from build123d import *

# Parameters (mm, degrees)
SKETCH_W        = 720
SKETCH_H        = 720
PAD_DEPTH       = 10
SKETCH001_W     = 700
SKETCH001_H     = 700
SKETCH001_W_2   = 680
SKETCH001_H_2   = 680
PAD001_DEPTH    = 50
SKETCH002_W     = 46
SKETCH002_H     = 40
SKETCH002_H_2   = 200
PAD002_DEPTH    = 10
SKETCH003_W     = 46
SKETCH003_H     = 61
PAD003_DEPTH    = 5
SKETCH004_W     = 132
SKETCH004_H     = 61
PAD004_DEPTH    = 46
POCKET_DEPTH    = 61
SKETCH006_R     = 2.5
PAD005_DEPTH    = 14
POCKET001_DEPTH = 10
SKETCH008_W     = 5
SKETCH008_H     = 83
SKETCH008_H_2   = 35
POCKET002_DEPTH = 10
FILLET_R        = 3
FILLET001_R     = 3
FILLET002_R     = 1
FILLET003_R     = 5
SKETCH009_W     = 80
SKETCH009_H     = 40
POCKET003_DEPTH = 10


with BuildPart() as part:
    # Sketch → Pad (new body)
    with BuildSketch(Plane.XY):
        Rectangle(SKETCH_W, SKETCH_H)
    extrude(amount=PAD_DEPTH)

    # Sketch001 (on Face5 of Pad) → Pad001 (join)
    with BuildSketch(Plane(origin=(0, 0, 0), x_dir=(1, 0, 0), z_dir=(0, 0, -1))):
        Rectangle(SKETCH001_W, SKETCH001_H)
        Rectangle(SKETCH001_W_2, SKETCH001_H_2, mode=Mode.SUBTRACT)
    extrude(amount=PAD001_DEPTH)

    # Sketch002 (on Face16 of Pad001) → Pad002 (join)
    with BuildSketch(Plane(origin=(0, 0, 0), x_dir=(1, 0, 0), z_dir=(0, 0, -1))):
        with Locations((282, -285)):
            Rectangle(SKETCH002_W, SKETCH002_H)
        with Locations((231, -285)):
            Rectangle(SKETCH002_W, SKETCH002_H)
        with Locations((282, -84)):
            Rectangle(SKETCH002_W, SKETCH002_H_2)
        with Locations((231, -84)):
            Rectangle(SKETCH002_W, SKETCH002_H_2)
    extrude(amount=PAD002_DEPTH)

    # Sketch003 (on Face16 of Pad002) → Pad003 (join)
    with BuildSketch(Plane(origin=(0, 0, 0), x_dir=(1, 0, 0), z_dir=(0, 0, -1))):
        with Locations((231, -224.5)):
            Rectangle(SKETCH003_W, SKETCH003_H)
        with Locations((282, -224.5)):
            Rectangle(SKETCH003_W, SKETCH003_H)
    extrude(amount=PAD003_DEPTH)

    # Sketch004 (on Face16 of Pad003) → Pad004 (join)
    with BuildSketch(Plane(origin=(0, 0, 0), x_dir=(1, 0, 0), z_dir=(0, 0, -1))):
        with Locations((-174, 209.5)):
            Rectangle(SKETCH004_W, SKETCH004_H)
    extrude(amount=PAD004_DEPTH)

    # Sketch005 (on Face42 of Pad004) → Pocket (cut)
    with BuildSketch(Plane(origin=(0, -179, 0), x_dir=(-1, 0, 0), z_dir=(0, 1, 0))):
        Polygon((108, -46), (240, -46), (179, 0), (169, 0), align=None)
    extrude(amount=-POCKET_DEPTH, mode=Mode.SUBTRACT)

    # Sketch006 (on Face16 of Pocket) → Pad005 (join)
    with BuildSketch(Plane(origin=(0, 0, 0), x_dir=(1, 0, 0), z_dir=(0, 0, -1))):
        with Locations((-241.5, -208.5)):
            Circle(SKETCH006_R)
    extrude(amount=PAD005_DEPTH)

    # Sketch007 (on Face13 of Pad005) → Pocket001 (cut)
    with BuildSketch(Plane.XZ.offset(-340)):
        with BuildLine():
            ThreePointArc((-292.75, -25), (-307.75, -10), (-322.75, -25))
            Line((-322.75, -50), (-322.75, -25))
            Line((-322.75, -50), (-292.75, -50))
            Line((-292.75, -50), (-292.75, -25))
        make_face()
    extrude(amount=-POCKET001_DEPTH, mode=Mode.SUBTRACT)

    # Sketch008 (on Face19 of Pocket001) → Pocket002 (cut)
    with BuildSketch(Plane(origin=(0, 0, 0), x_dir=(1, 0, 0), z_dir=(0, 0, -1))):
        with Locations((-286.5, -208.5)):
            Rectangle(SKETCH008_W, SKETCH008_H)
        with Locations((-279, -208.5)):
            Rectangle(SKETCH008_W, SKETCH008_H)
        with Locations((-271.5, -208.5)):
            Rectangle(SKETCH008_W, SKETCH008_H)
        with Locations((-264, -208.5)):
            Rectangle(SKETCH008_W, SKETCH008_H)
        with Locations((-256.5, -208.5)):
            Rectangle(SKETCH008_W, SKETCH008_H)
        with Locations((-249, -208.5)):
            Rectangle(SKETCH008_W, SKETCH008_H)
        with Locations((-234, -208.5)):
            Rectangle(SKETCH008_W, SKETCH008_H)
        with Locations((-226.5, -208.5)):
            Rectangle(SKETCH008_W, SKETCH008_H)
        with Locations((-241.5, -184.5)):
            Rectangle(SKETCH008_W, SKETCH008_H_2)
        with Locations((-241.5, -232.5)):
            Rectangle(SKETCH008_W, SKETCH008_H_2)
        with Locations((-219, -208.5)):
            Rectangle(SKETCH008_W, SKETCH008_H)
        with Locations((-211.5, -208.5)):
            Rectangle(SKETCH008_W, SKETCH008_H)
        with Locations((-204, -208.5)):
            Rectangle(SKETCH008_W, SKETCH008_H)
        with Locations((-196.5, -208.5)):
            Rectangle(SKETCH008_W, SKETCH008_H)
        with Locations((-294, -208.5)):
            Rectangle(SKETCH008_W, SKETCH008_H)
        with Locations((-189, -208.5)):
            Rectangle(SKETCH008_W, SKETCH008_H)
    extrude(amount=-POCKET002_DEPTH, mode=Mode.SUBTRACT)

    # Fillet
    fillet_edges = [part.edges().sort_by_distance(p)[0] for p in [
        (-307.75, 340, -10),
        (-307.75, 350, -10),
        (-322.75, 340, -37.5),
        (-292.75, 340, -37.5),
        (-292.75, 350, -37.5),
        (-322.75, 350, -37.5),
    ]]
    fillet(fillet_edges, radius=FILLET_R)

    # Fillet001
    fillet001_edges = [part.edges().sort_by_distance(p)[0] for p in [
        (208, 285, -10),
        (231, 305, -10),
        (231, 265, -10),
        (254, 285, -10),
        (259, 285, -10),
        (282, 305, -10),
        (282, 265, -10),
        (305, 285, -10),
        (305, 224.5, -5),
        (282, 255, -5),
        (259, 224.5, -5),
        (282, 194, -5),
        (254, 224.5, -5),
        (231, 255, -5),
        (208, 224.5, -5),
        (231, 194, -5),
        (208, 84, -10),
        (231, 184, -10),
        (254, 84, -10),
        (231, -16, -10),
        (259, 84, -10),
        (282, -16, -10),
        (305, 84, -10),
        (282, 184, -10),
    ]]
    fillet(fillet001_edges, radius=FILLET001_R)

    # Fillet002
    fillet002_edges = [part.edges().sort_by_distance(p)[0] for p in [
        (-209.5, -179, -23),
        (-209.5, -240, -23),
        (-138.5, -179, -23),
        (-138.5, -240, -23),
        (-240, -209.5, -46),
        (-108, -209.5, -46),
    ]]
    fillet(fillet002_edges, radius=FILLET002_R)

    # Fillet003
    fillet003_edges = [part.edges().sort_by_distance(p)[0] for p in [
        (-360, 0, 10),
        (0, -360, 10),
        (-360, -360, 5),
        (-360, 360, 5),
        (0, 360, 10),
        (360, 360, 5),
        (360, 0, 10),
        (360, -360, 5),
    ]]
    fillet(fillet003_edges, radius=FILLET003_R)

    # Sketch009 (on Face123 of Fillet003) → Pocket003 (cut)
    with BuildSketch(Plane.XZ.offset(350)):
        with Locations((-280, -30)):
            Rectangle(SKETCH009_W, SKETCH009_H)
    extrude(amount=-POCKET003_DEPTH, mode=Mode.SUBTRACT)


solid = part.part
Could you check a few things on this model? Use its own coordinates, in mm. A direction names the side the tool comes from. Give positions to 0.01 mm unless a question says otherwise; leave off trailing zeros. Write each loop counter-clockwise with the first axis right and the second up, starting at its lowest first coordinate (ties: lowest second). Pieces come first, ordered by that corner, then holes. Notation, with made-up numbers: (76, 48) -> (94, 48) arc R16 ccw to (94, 54) -> close; hole circle Ø4 at (64.25, 35.25). An arc over 180 degrees is marked (long way). Write each question's results on one line, items separated by ' | '. Start each with the question number.
Q1. Suppose I cut it at B-B, the plane y = -97.5. List the corners of the cut face in (x, z) for me.
Q2. I'm going to push flat-ended pins straight in: pin 1 Ø7.5 at (x, z) = (284.5, -3.5) entering from -Y; pin 2 Ø1.5 at (x, z) = (96, -39.5) entering from +Y; pin 3 Ø5 at (y, z) = (-8.5, -41.5) entering from -X; pin 4 Ø15 at (y, z) = (57.5, -27.5) entering from +X. Where does each tip first touch, or does it pass through?
Q3. We'd pull the mould along X, two halves only. Please class faces 3 (the face through (-5, 350, -25)), 4 (the face through (350, 5, -25)), 5 (the face through (-5, 340, -25)): +X half, -X half, draft (parallel to the pull), parting line (faces both ways), or undercut.
Q4. Suppose I cut it at A-A, the plane x = -307.75. List the corners of the cut face in (y, z) for me, and give its area (3 significant figures).
Q5. I need wall thicknesses on probe 1 along X at (y, z) = (267, -8); probe 2 along Y at (x, z) = (-223.5, -36.5); probe 3 along X at (y, z) = (102, -0.5). Which ranges of each line are inside material? Lowest first, please.
Q6. Which directions (+Z, -Z, +X, -X, +Y, -Y) give clear straight access to the entire face, cutting with the end or side of a thin tool? Please do faces 1 (the face through (-217, -179, -17)), 2 (the face through (-5, 5, 10)).
Outcome:
1) outline: (-360, 0) -> (-350, 0) -> (-350, -50) -> (-340, -50) -> (-340, 0) -> (340, 0) -> (340, -50) -> (350, -50) -> (350, 0) -> (360, 0) -> (360, 5) arc R5 ccw to (355, 10) -> (-355, 10) arc R5 ccw to (-360, 5) -> close
2) pin 1: y = -360 | pin 2: y = 350 | pin 3: x = -350 | pin 4: x = 350
3) face 3: draft | face 4: +X half | face 5: undercut
4) outline: (-360, 0) -> (-350, 0) -> (-350, -10) -> (-340, -10) -> (-340, 0) -> (340, 0) -> (340, -7) arc R3 ccw to (343, -10) -> (347, -10) arc R3 ccw to (350, -7) -> (350, 0) -> (360, 0) -> (360, 5) arc R5 ccw to (355, 10) -> (-355, 10) arc R5 ccw to (-360, 5) -> close | area: 7,390 mm2
5) probe 1: -350 to -340, 208.17 to 253.83, 259.17 to 304.83, 340 to 350 | probe 2: -350 to -340, 340 to 350 | probe 3: -350 to -340, 208 to 254, 259 to 305, 340 to 350
6) face 1: -Z | face 2: +Z, +X, -X, +Y, -Y
